Geometry: final body of the model. Coordinates: model frame, mm. A direction names the side the tool comes from. Give positions to 0.01 mm unless a question says otherwise; leave off trailing zeros. Order: outer loops, then holes, each group sorted by start corner. A loop starts at its lowest first (then second) coordinate and runs counter-clockwise, first axis right, second up. Notation, with made-up numbers: (48.25, -10.75) - (88.25, -10.75) arc R19 ccw to (88.25, -3.75) - close; hole circle Ø10 at (18.5, -30). An arc over 180 degrees is marked (long way). Put each result on its own line as item: value. Start each with the question number.
1. Ray query, line 1 along X through (y, z) = (24, -12.5); line 2 along Z through (x, y) = (27.5, 42); line 3 along Y through (x, z) = (57.65, 11.5). Return the intervals inside material, ascending. Write a range as from..to.
2. Section D-D on x = -3.5. Return the cut outline in (y, z).
3. Mould query, pull axis X, two halves, no side actions, for faces 4 (the cylindrical face through (-57.9, 83.4, 11.1)), 5 (the flat face through (-1, 28, 25.3)), 6 (the flat face through (57, 47, 0)), 7 (the flat face through (58.8, 46, 0)). Classes: pulls with the +X half, pulls with the -X half, needs draft (parallel to the pull), parting line crosses it, or undercut.
4. Set-up query: faces 1 (the cylindrical face through (45.624, 13.041, -26.213)), 2 (the flat face through (-1, 3, 0)), 3 (the cylindrical face through (25, 17, 26)). Return all of +Z, -Z, +X, -X, +Y, -Y with unobstructed straight access to the full face (end or side cutting, diameter ignored); none if empty.
5. Section A-A on y = 85. Return the cut outline in (x, z).
6. Section B-B on x = -27.5. Return the cut outline in (y, z).
7. First-contact query: P1, Ø15, axis at x = 10, z = -11.5, coming from the +Y side; P2, Ø2, axis at x = 2.575, y = 14.075, coming from the -Z side; P3, Ø1.4, axis at x = 58, y = 63.5, coming from the +Z side. Flat tips, straight axial feed; report the tip coordinate or a pass-through.
8. Section C-C on z = 11.5. Return the cut outline in (x, y).
from build123d import *

# Parameters (mm, degrees)
SKETCH2_W           = 117.6
SKETCH2_H           = 54.2
BOSS_EXTRUDE1_DEPTH = 3
SKETCH3_W           = 117.6
SKETCH3_H           = 54.2
SKETCH3_W_2         = 114
SKETCH3_H_2         = 50.6
BOSS_EXTRUDE2_DEPTH = 50
BOSS_EXTRUDE3_DEPTH = 40
CHAMFER1_SIZE       = 10
SKETCH5_R           = 1.65
CUT_EXTRUDE1_DEPTH  = 153.358688627
CUT_EXTRUDE2_REACH  = 124.654
SKETCH6_R           = 1.7
SKETCH6_W           = 28
SKETCH6_H           = 19.6
SKETCH6_H_2         = 22
CUT_EXTRUDE3_REACH  = 124.654


with BuildPart() as part:
    # Sketch2 → Boss-Extrude1 (new body)
    with BuildSketch(Plane(origin=(0, 0, 0), x_dir=(1, 0, 0), z_dir=(0, 1, 0))):
        Rectangle(SKETCH2_W, SKETCH2_H)
    extrude(amount=BOSS_EXTRUDE1_DEPTH)

    # Sketch3 → Boss-Extrude2 (add)
    with BuildSketch(Plane(origin=(0, 3, 0), x_dir=(1, 0, 0), z_dir=(0, 1, 0))):
        Rectangle(SKETCH3_W, SKETCH3_H)
        Rectangle(SKETCH3_W_2, SKETCH3_H_2, mode=Mode.SUBTRACT)
    extrude(amount=BOSS_EXTRUDE2_DEPTH)

    # Sketch4 → Boss-Extrude3 (add)
    with BuildSketch(Plane(origin=(0, 53, 0), x_dir=(1, 0, 0), z_dir=(0, 1, 0))):
        Polygon((57, -25.3), (57, 25.3), (-57, 25.3), (-57, -25.3), (-58.8, -25.3), (-58.8, 27.1), (58.8, 27.1), (58.8, -25.3), align=None)
    extrude(amount=BOSS_EXTRUDE3_DEPTH)

    # Chamfer1
    chamfer1_edges = [part.edges().sort_by_distance(p)[0] for p in [
        (-57.9, 93, 25.3),
        (57.9, 93, 25.3),
    ]]
    chamfer(chamfer1_edges, length=CHAMFER1_SIZE)

    # Sketch5 → Cut-Extrude1 (cut, through all)
    with BuildSketch(Plane.ZY.offset(58.8)):
        with Locations((11.5, 85)):
            Circle(SKETCH5_R)
        with Locations((-13.5, 85)):
            Circle(SKETCH5_R)
    extrude(amount=-CUT_EXTRUDE1_DEPTH, mode=Mode.SUBTRACT)

    # Sketch6 → Cut-Extrude2 (cut, up to next)
    with BuildSketch(Plane(origin=(0, 0, -27.1), x_dir=(-1, 0, 0), z_dir=(0, 0, -1)), mode=Mode.PRIVATE) as cut_extrude2_sk1:
        with Locations((-2.575, 14.075)):
            Circle(SKETCH6_R)
    cut_extrude2_tool1 = extrude(cut_extrude2_sk1.sketch, amount=-CUT_EXTRUDE2_REACH, mode=Mode.PRIVATE) & part.part
    # Sketch6 → Cut-Extrude2 (cut, up to next)
    with BuildSketch(Plane(origin=(0, 0, -27.1), x_dir=(-1, 0, 0), z_dir=(0, 0, -1)), mode=Mode.PRIVATE) as cut_extrude2_sk2:
        with Locations((-44.275, 14.075)):
            Circle(SKETCH6_R)
    cut_extrude2_tool2 = extrude(cut_extrude2_sk2.sketch, amount=-CUT_EXTRUDE2_REACH, mode=Mode.PRIVATE) & part.part
    # Sketch6 → Cut-Extrude2 (cut, up to next)
    with BuildSketch(Plane(origin=(0, 0, -27.1), x_dir=(-1, 0, 0), z_dir=(0, 0, -1)), mode=Mode.PRIVATE) as cut_extrude2_sk3:
        with Locations((-25.4, 14)):
            Rectangle(SKETCH6_W, SKETCH6_H)
    cut_extrude2_tool3 = extrude(cut_extrude2_sk3.sketch, amount=-CUT_EXTRUDE2_REACH, mode=Mode.PRIVATE) & part.part
    # Sketch6 → Cut-Extrude2 (cut, up to next)
    with BuildSketch(Plane(origin=(0, 0, -27.1), x_dir=(-1, 0, 0), z_dir=(0, 0, -1)), mode=Mode.PRIVATE) as cut_extrude2_sk4:
        with Locations((30.5, 15.8)):
            Rectangle(SKETCH6_W, SKETCH6_H_2)
    cut_extrude2_tool4 = extrude(cut_extrude2_sk4.sketch, amount=-CUT_EXTRUDE2_REACH, mode=Mode.PRIVATE) & part.part
    add(cut_extrude2_tool1.solids().sort_by_distance((2.575, 14.075, -27.1))[0], mode=Mode.SUBTRACT)
    add(cut_extrude2_tool2.solids().sort_by_distance((44.275, 14.075, -27.1))[0], mode=Mode.SUBTRACT)
    add(cut_extrude2_tool3.solids().sort_by_distance((25.4, 14, -27.1))[0], mode=Mode.SUBTRACT)
    add(cut_extrude2_tool4.solids().sort_by_distance((-30.5, 15.8, -27.1))[0], mode=Mode.SUBTRACT)

    # Sketch7 → Cut-Extrude3 (cut, up to next)
    with BuildSketch(Plane.XY.offset(27.1), mode=Mode.PRIVATE) as cut_extrude3_sk1:
        with BuildLine():
            Line((22, 6), (22, 14))
            ThreePointArc((22, 14), (25, 17), (28, 14))
            Line((28, 14), (28, 6))
            ThreePointArc((28, 6), (25, 3), (22, 6))
        make_face()
    cut_extrude3_tool1 = extrude(cut_extrude3_sk1.sketch, amount=-CUT_EXTRUDE3_REACH, mode=Mode.PRIVATE) & part.part
    add(cut_extrude3_tool1.solids().sort_by_distance((25, 10, 27.1))[0], mode=Mode.SUBTRACT)


solid = part.part
Resolved:
1. line 1: -58.8..-57, 57..58.8
1. line 2: -27.1..-25.3, 25.3..27.1
1. line 3: 0..83.35, 86.65..93
2. outline: (0, -27.1) - (93, -27.1) - (93, -25.3) - (3, -25.3) - (3, 25.3) - (53, 25.3) - (53, 27.1) - (0, 27.1) - close
3. face 4: needs draft
3. face 5: undercut
3. face 6: undercut
3. face 7: pulls with the +X half
4. face 1: -Z
4. face 2: +Y
4. face 3: +Z, -Z
5. outline: (-58.8, -27.1) - (58.8, -27.1) - (58.8, -15.15) - (57, -15.15) - (57, -25.3) - (-57, -25.3) - (-57, -15.15) - (-58.8, -15.15) - close; (-58.8, -11.85) - (-57, -11.85) - (-57, 9.85) - (-58.8, 9.85) - close; (-58.8, 13.15) - (-57, 13.15) - (-57, 23.3) - (-58.8, 23.3) - close; (57, -11.85) - (58.8, -11.85) - (58.8, 9.85) - (57, 9.85) - close; (57, 13.15) - (58.8, 13.15) - (58.8, 23.3) - (57, 23.3) - close
6. outline: (0, -27.1) - (4.8, -27.1) - (4.8, -25.3) - (3, -25.3) - (3, 25.3) - (53, 25.3) - (53, 27.1) - (0, 27.1) - close; (26.8, -27.1) - (93, -27.1) - (93, -25.3) - (26.8, -25.3) - close
7. P1: y = 3
7. P2: z = 25.3
7. P3: z = 25.3
8. outline: (-58.8, 0) - (58.8, 0) - (58.8, 83.35) - (57, 83.35) - (57, 3) - (-57, 3) - (-57, 83.35) - (-58.8, 83.35) - close; (-58.8, 86.65) - (-57, 86.65) - (-57, 93) - (-58.8, 93) - close; (57, 86.65) - (58.8, 86.65) - (58.8, 93) - (57, 93) - close
